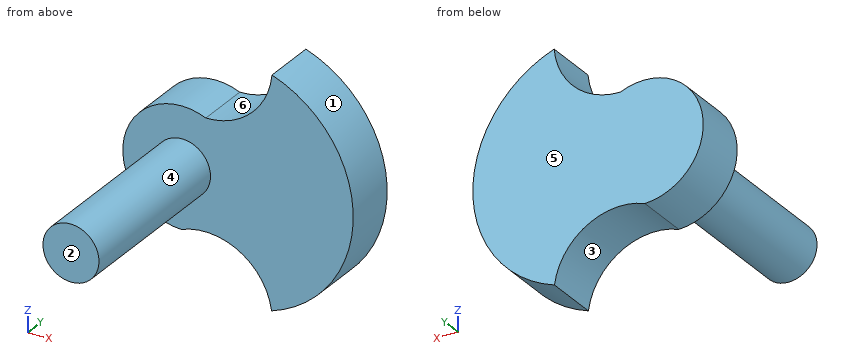
```python
from build123d import *

# Parameters (mm, degrees)
F0_R     = 5.9055
F1_DEPTH = 11.43
F2_DEPTH = 48.9966


with BuildPart() as f1:
    # F0 (on Front) → F1 (new body)
    with BuildSketch(Plane.XZ):
        with BuildLine():
            ThreePointArc((-5.19436, -10.830459), (7.032524, -11.726022), (13.86311, -21.906485))
            ThreePointArc((13.86311, -21.906485), (31.07098, 2.06154), (13.941479, 26.085635))
            ThreePointArc((13.941479, 26.085635), (9.452353, 16.991928), (0, 13.317586))
            ThreePointArc((0, 13.317586), (-17.216361, 4.38822), (-5.19436, -10.830459))
        make_face()
        with Locations((-4.920786, 1.743383)):
            Circle(F0_R, mode=Mode.SUBTRACT)
    extrude(amount=F1_DEPTH)

    # F0 (on Front) → F2 (join)
    with BuildSketch(Plane.XZ):
        with Locations((-4.920786, 1.743383)):
            Circle(F0_R)
    extrude(amount=F2_DEPTH)


solid = f1.part
```
Read the model definition and answer for the solid it produces. Units are mm, in the model's axes. Face numbers are marked on the shaded views. A direction names the side the tool comes from. Give positions to 0.01 mm unless a question says otherwise; leave off trailing zeros. Order: outer loops, then holes, each group sorted by start corner. A loop starts at its lowest first (then second) coordinate and runs counter-clockwise, first axis right, second up.
(1) Find section A-A (z = 2.5). Give the vertices of the cut face in (x, y).
(2) For the marked faces 4, 5 and 6, determine the directions among +Z, -Z, +X, -X, +Y, -Y from which every point of the face is accessible in a straight line to the end or side of a thin tool.
(3) Find section D-D (z = -5). Give the vertices of the cut face in (x, y), plus the area to 3 significant figures.
(4) Given pin 1 (14.5 mm diameter, centred on x = 3, z = 13.5, fed in from -Y); pin 2 (1 mm diameter, centred on y = -41, z = 6, fed in from +X); pin 3 (4 mm diameter, centred on y = -41.5, z = 4, fed in from -X), each flat-ended and moving along its own axis, determine where each tip first touches the part or whether it passes through.
(5) For a pull along Z with two mould halves and no side action, classify the marked faces 1, 2 and 3 as released by +Z, released by -Z, zero draft, split by the parting line, or undercut.
(6) Find section C-C (y = -32.5). Give the vertices of the cut face in (x, z).
(7) Find section B-B (x = -1.5). Give the vertices of the cut face in (y, z).
(8) Straight lines are drawn through the part: L1, parallel to Z at x = -5, y = -41.5; L2, parallel to Y at x = 16, z = 8.5; L3, parallel to Z at x = -7, y = -10.5. For each, find the intervals that lie inside material, in ascending order.
Result sheet:
1. outline: (-17.47, -11.43) - (-10.78, -11.43) - (-10.78, -49) - (0.94, -49) - (0.94, -11.43) - (31.07, -11.43) - (31.07, 0) - (-17.47, 0) - close
2. face 4: -Y
2. face 5: +Z, -Z, +X, -X, +Y
2. face 6: +Z, +Y, -Y
3. outline: (-15.54, -11.43) - (30.06, -11.43) - (30.06, 0) - (-15.54, 0) - close
3. area: 521 mm2
4. pin 1: stops at y = -11.43
4. pin 2: stops at x = -0.36
4. pin 3: stops at x = -10.82
5. face 1: split by the parting line
5. face 2: zero draft
5. face 3: released by -Z
6. outline: circle Ø11.81 at (-4.92, 1.74)
7. outline: (-49, -3.07) - (-11.43, -3.07) - (-11.43, -9.91) - (0, -9.91) - (0, 13.85) - (-11.43, 13.85) - (-11.43, 6.56) - (-49, 6.56) - close
8. L1: z = -4.16 to 7.65
8. L2: y = -11.43 to 0
8. L3: z = -10.66 to 14.15
